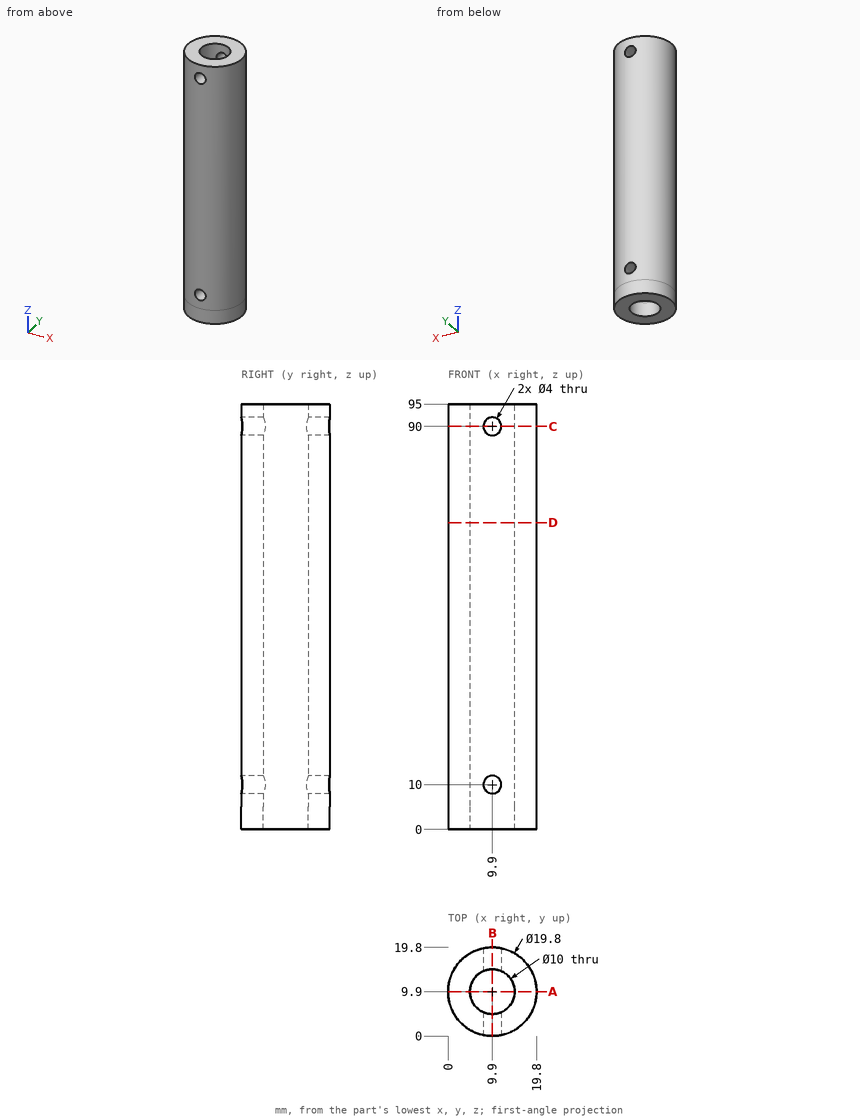
Design review of the part shown in the three views and the two pictorial views. Dimensions are in mm from the part's minimum x, y and z. Give positions to 0.01 mm unless a question says otherwise; leave off trailing zeros. Loops run counter-clockwise (first coordinate to the right, second up) from the corner with the lowest first, then second, coordinate; pieces in that order, holes last. Notation, with made-up numbers: M 20.5,1.25 L 61.5,1.25 A15 cw 61.5,10.25 Z; hole C 4,86.25 d4. An arc over 180 degrees is marked long. Answer as a JSON object with one key per item and string values.
Item 1: We need section B-B (x = 9.9). State the section outline as (y, z) points.
Output values:
{"outline": "M 0,0 L 4.9,0 L 4.9,8 L 0,8 Z; M 0,12 L 4.9,12 L 4.9,88 L 0,88 Z; M 0,92 L 4.9,92 L 4.9,95 L 0,95 Z; M 14.9,0 L 19.8,0 L 19.8,8 L 14.9,8 Z; M 14.9,12 L 19.8,12 L 19.8,88 L 14.9,88 Z; M 14.9,92 L 19.8,92 L 19.8,95 L 14.9,95 Z"}
Item 2: We need section D-D (z = 68.5). State the section outline as (x, y) points.
Output values:
{"outline": "C 9.9,9.9 d19.8; hole C 9.9,9.9 d10"}
Item 3: For P1, Ø2, axis at y = 4, z = 30.5, coming from the +X side; P2, Ø4.5, axis at x = 9.9, z = 90, coming from the +Y side; P3, Ø5, axis at x = 16.5, z = 42.5, coming from the -Y side; P4, Ø3, axis at x = 9.9, z = 90, coming from the -Y side (3 decimals), all flat-tipped, find the tip position at first contact; note any pin that passes through.
Output values:
{"P1": "stops at x = 18.5", "P2": "stops at y = 19.8", "P3": "stops at y = 0.89", "P4": "passes through"}
Item 4: We need section A-A (y = 9.9). State the section outline as (x, z) points.
Output values:
{"outline": "M 0,0 L 4.9,0 L 4.9,95 L 0,95 Z; M 14.9,0 L 19.8,0 L 19.8,95 L 14.9,95 Z"}
Item 5: We need section C-C (z = 90). State the section outline as (x, y) points, and give its area (3 significant figures).
Output values:
{"outline": "M 7.9,0.2 L 7.9,5.32 A5 cw 7.9,14.48 L 7.9,19.6 A9.9 ccw Z; M 11.9,0.2 A9.9 ccw 11.9,19.6 L 11.9,14.48 A5 cw 11.9,5.32 Z", "area": "190 mm2"}
Item 6: Wall thickness on line 1 along Y through (x, z) = (10, 74.5); line 2 along X through (y, z) = (10.25, 17); line 3 along Y through (x, z) = (6, 14.5): over which ranges is each line inside the solid? List them lowest first.
Output values:
{"line 1": "y = 0 to 4.9, 14.9 to 19.8", "line 2": "x = 0.01 to 4.91, 14.89 to 19.79", "line 3": "y = 0.8 to 6.77, 13.03 to 19"}
